Design review of the part built by this model. Coordinates are the model's own, in mm. A direction names the side the tool comes from. Coordinates: 2 decimals unless noted, no trailing zeros. Use a Markdown table: item, result.
from build123d import *

# Parameters (mm, degrees)
F0_R     = 11.1
F0_R_2   = 7
F1_DEPTH = 0.6
F2_DEPTH = 8.5
F3_R     = 11.8527911282
F4_SIZE  = 0.8
F5_DEPTH = 1.3


# Not quite as in the source:
# - a feature names something its author has since deleted; it is built from what else it names


with BuildPart() as f1:
    # F0 (on Top) → F1 (new body)
    with BuildSketch(Plane.XY):
        with BuildLine():
            ThreePointArc((-3.5707142143, 12.5), (0, 13), (3.5707142143, 12.5))
            ThreePointArc((3.5707142143, 12.5), (10.3783256064, 17.1711841504), (13, 25))
            ThreePointArc((13, 25), (-7.8288158496, 35.3783256064), (-3.5707142143, 12.5))
        make_face()
        Polygon((4.9074772881, 33.5), (9.8149545762, 25), (4.9074772881, 16.5), (-4.9074772881, 16.5), (-9.8149545762, 25), (-4.9074772881, 33.5), align=None, mode=Mode.SUBTRACT)
        with BuildLine():
            ThreePointArc((-9.0399604402, -9.3423292192), (-11.2583302492, -6.5), (-12.6106746544, -3.1576707808))
            ThreePointArc((-12.6106746544, -3.1576707808), (-33.6197513051, -17.5734856991), (-8.6506350946, -12.5))
            ThreePointArc((-8.6506350946, -12.5), (-8.7483335459, -10.9092093959), (-9.0399604402, -9.3423292192))
        make_face()
        Polygon((-26.5581123827, -4), (-16.7431578065, -4), (-11.8356805184, -12.5), (-16.7431578065, -21), (-26.5581123827, -21), (-31.4655896708, -12.5), align=None, mode=Mode.SUBTRACT)
        with BuildLine():
            ThreePointArc((34.6506350946, -12.5), (26.7241207937, -0.5308837895), (12.6106746544, -3.1576707808))
            ThreePointArc((12.6106746544, -3.1576707808), (11.2583302492, -6.5), (9.0399604402, -9.3423292192))
            ThreePointArc((9.0399604402, -9.3423292192), (20.0598444905, -25.4023015487), (34.6506350946, -12.5))
        make_face()
        Polygon((16.7431578065, -21), (11.8356805184, -12.5), (16.7431578065, -4), (26.5581123827, -4), (31.4655896708, -12.5), (26.5581123827, -21), align=None, mode=Mode.SUBTRACT)
        with BuildLine():
            ThreePointArc((12.6106746544, -3.1576707808), (12.9023015487, -1.5907906041), (13, 0))
            ThreePointArc((13, 0), (10.3783256064, 7.8288158496), (3.5707142143, 12.5))
            ThreePointArc((3.5707142143, 12.5), (0, 12), (-3.5707142143, 12.5))
            ThreePointArc((-3.5707142143, 12.5), (-11.2583302492, 6.5), (-12.6106746544, -3.1576707808))
            ThreePointArc((-12.6106746544, -3.1576707808), (-10.3923048454, -6), (-9.0399604402, -9.3423292192))
            ThreePointArc((-9.0399604402, -9.3423292192), (0, -13), (9.0399604402, -9.3423292192))
            ThreePointArc((9.0399604402, -9.3423292192), (10.3923048454, -6), (12.6106746544, -3.1576707808))
        make_face()
        Circle(F0_R, mode=Mode.SUBTRACT)
        Circle(F0_R)
        Circle(F0_R_2, mode=Mode.SUBTRACT)
        Polygon((4.9074772881, 16.5), (9.8149545762, 25), (4.9074772881, 33.5), (-4.9074772881, 33.5), (-9.8149545762, 25), (-4.9074772881, 16.5), align=None)
        Polygon((-11.8356805184, -12.5), (-16.7431578065, -4), (-26.5581123827, -4), (-31.4655896708, -12.5), (-26.5581123827, -21), (-16.7431578065, -21), align=None)
        Polygon((16.7431578065, -4), (11.8356805184, -12.5), (16.7431578065, -21), (26.5581123827, -21), (31.4655896708, -12.5), (26.5581123827, -4), align=None)
        with BuildLine():
            ThreePointArc((-3.5707142143, 12.5), (0, 12), (3.5707142143, 12.5))
            ThreePointArc((3.5707142143, 12.5), (0, 13), (-3.5707142143, 12.5))
        make_face()
        with BuildLine():
            ThreePointArc((-9.0399604402, -9.3423292192), (-10.3923048454, -6), (-12.6106746544, -3.1576707808))
            ThreePointArc((-12.6106746544, -3.1576707808), (-11.2583302492, -6.5), (-9.0399604402, -9.3423292192))
        make_face()
        with BuildLine():
            ThreePointArc((9.0399604402, -9.3423292192), (11.2583302492, -6.5), (12.6106746544, -3.1576707808))
            ThreePointArc((12.6106746544, -3.1576707808), (10.3923048454, -6), (9.0399604402, -9.3423292192))
        make_face()
    extrude(amount=F1_DEPTH)

    # F0 (on Top) → F2 (join)
    with BuildSketch(Plane.XY):
        with BuildLine():
            ThreePointArc((-3.5707142143, 12.5), (0, 13), (3.5707142143, 12.5))
            ThreePointArc((3.5707142143, 12.5), (10.3783256064, 17.1711841504), (13, 25))
            ThreePointArc((13, 25), (-7.8288158496, 35.3783256064), (-3.5707142143, 12.5))
        make_face()
        Polygon((4.9074772881, 33.5), (9.8149545762, 25), (4.9074772881, 16.5), (-4.9074772881, 16.5), (-9.8149545762, 25), (-4.9074772881, 33.5), align=None, mode=Mode.SUBTRACT)
        with BuildLine():
            ThreePointArc((12.6106746544, -3.1576707808), (12.9023015487, -1.5907906041), (13, 0))
            ThreePointArc((13, 0), (10.3783256064, 7.8288158496), (3.5707142143, 12.5))
            ThreePointArc((3.5707142143, 12.5), (0, 12), (-3.5707142143, 12.5))
            ThreePointArc((-3.5707142143, 12.5), (-11.2583302492, 6.5), (-12.6106746544, -3.1576707808))
            ThreePointArc((-12.6106746544, -3.1576707808), (-10.3923048454, -6), (-9.0399604402, -9.3423292192))
            ThreePointArc((-9.0399604402, -9.3423292192), (0, -13), (9.0399604402, -9.3423292192))
            ThreePointArc((9.0399604402, -9.3423292192), (10.3923048454, -6), (12.6106746544, -3.1576707808))
        make_face()
        Circle(F0_R, mode=Mode.SUBTRACT)
        with BuildLine():
            ThreePointArc((-3.5707142143, 12.5), (0, 12), (3.5707142143, 12.5))
            ThreePointArc((3.5707142143, 12.5), (0, 13), (-3.5707142143, 12.5))
        make_face()
        with BuildLine():
            ThreePointArc((-9.0399604402, -9.3423292192), (-11.2583302492, -6.5), (-12.6106746544, -3.1576707808))
            ThreePointArc((-12.6106746544, -3.1576707808), (-33.6197513051, -17.5734856991), (-8.6506350946, -12.5))
            ThreePointArc((-8.6506350946, -12.5), (-8.7483335459, -10.9092093959), (-9.0399604402, -9.3423292192))
        make_face()
        Polygon((-26.5581123827, -4), (-16.7431578065, -4), (-11.8356805184, -12.5), (-16.7431578065, -21), (-26.5581123827, -21), (-31.4655896708, -12.5), align=None, mode=Mode.SUBTRACT)
        with BuildLine():
            ThreePointArc((-9.0399604402, -9.3423292192), (-10.3923048454, -6), (-12.6106746544, -3.1576707808))
            ThreePointArc((-12.6106746544, -3.1576707808), (-11.2583302492, -6.5), (-9.0399604402, -9.3423292192))
        make_face()
        with BuildLine():
            ThreePointArc((34.6506350946, -12.5), (26.7241207937, -0.5308837895), (12.6106746544, -3.1576707808))
            ThreePointArc((12.6106746544, -3.1576707808), (11.2583302492, -6.5), (9.0399604402, -9.3423292192))
            ThreePointArc((9.0399604402, -9.3423292192), (20.0598444905, -25.4023015487), (34.6506350946, -12.5))
        make_face()
        Polygon((16.7431578065, -21), (11.8356805184, -12.5), (16.7431578065, -4), (26.5581123827, -4), (31.4655896708, -12.5), (26.5581123827, -21), align=None, mode=Mode.SUBTRACT)
        with BuildLine():
            ThreePointArc((9.0399604402, -9.3423292192), (11.2583302492, -6.5), (12.6106746544, -3.1576707808))
            ThreePointArc((12.6106746544, -3.1576707808), (10.3923048454, -6), (9.0399604402, -9.3423292192))
        make_face()
    extrude(amount=F2_DEPTH)

    # F3
    f3_edges = [f1.edges().sort_by_distance(p)[0] for p in [
        (3.570714, 12.5, 4.25),
        (-3.570714, 12.5, 4.25),
        (-12.610675, -3.157671, 4.25),
        (-9.03996, -9.342329, 4.25),
        (9.03996, -9.342329, 4.25),
        (12.610675, -3.157671, 4.25),
    ]]
    fillet(f3_edges, radius=F3_R)

    # F4
    f4_edges = [f1.edges().sort_by_distance(p)[0] for p in [
        (11.25833, 6.5, 8.5),
        (9.627694, 12.5, 8.5),
        (0, 38, 8.5),
        (-9.627694, 12.5, 8.5),
        (-11.25833, 6.5, 8.5),
        (-11.25833, 6.5, 0),
        (-9.627694, 12.5, 0),
        (0, 38, 0),
        (9.627694, 12.5, 0),
        (11.25833, 6.5, 0),
        (15.639164, 2.087827, 8.5),
        (-15.639164, 2.087827, 8.5),
        (32.908965, -19, 8.5),
        (-32.908965, -19, 8.5),
        (6.011471, -14.587827, 8.5),
        (-6.011471, -14.587827, 8.5),
        (0, -13, 8.5),
        (15.639164, 2.087827, 0),
        (-15.639164, 2.087827, 0),
        (32.908965, -19, 0),
        (-32.908965, -19, 0),
        (6.011471, -14.587827, 0),
        (-6.011471, -14.587827, 0),
        (0, -13, 0),
    ]]
    chamfer(f4_edges, length=F4_SIZE)

    # F0 (on Top) → F5 (join)
    with BuildSketch(Plane.XY):
        Circle(F0_R)
        Circle(F0_R_2, mode=Mode.SUBTRACT)
    extrude(amount=F5_DEPTH)


solid = f1.part
(1) For pin 1 (4 mm diameter, centred on x = 21, z = 3, fed in from +Y); pin 2 (4 mm diameter, centred on x = -19.5, z = 4, fed in from +Y); pin 3 (11 mm diameter, centred on x = -3.5, y = -1, fed in from +Z), all flat-tipped, find the tip position at first contact; note any pin that passes through.
Determined:
| item | result |
|---|---|
| pin 1 | y = 0.78 |
| pin 2 | y = 1.22 |
| pin 3 | z = 1.3 |
(2) Machinability: for faces 3 (the flat face through (-29.046, -8.31, 4.495)), 4 (the conical face through (0.362, 37.334, 0.139)), which of the approach directions +Z, -Z, +X, -X, +Y, -Y give a long, thin tool a straight path to every point of the face, cutting with its end or side? Answer none if there is none.
Determined:
| item | result |
|---|---|
| face 3 | +Z |
| face 4 | -Z |
(3) Draft analysis for pull direction Y (two halves, no side actions). For faces 1 (the conical face through (-32.513, -18.353, 0.139)), 2 (the flat face through (-28.977, -16.81, 4.495)), state which applies: +Y half, -Y half, draft (parallel to the pull), parting line (faces both ways), or undercut.
Determined:
| item | result |
|---|---|
| face 1 | parting line |
| face 2 | undercut |
(4) Take a section at A-A on z = 6.5. State how many separate pieces and enclosed holes the cut face has, and give its area (3 significant figures).
Determined:
| item | result |
|---|---|
| separate pieces | 1 |
| enclosed holes | 4 |
| area | 1,090 mm2 |
(5) For L1, parallel to Y at x = 0, z = 1.05; L2, parallel to Y at x = 0, z = 7; L3, parallel to X at y = -20.5, z = 5, list the stretches that pass through material, from the lowest coordinate up. Write a range as from..to.
Determined:
| item | result |
|---|---|
| L1 | -13..-7, 7..16.5, 33.5..38 |
| L2 | -13..-11.1, 11.1..16.5, 33.5..38 |
| L3 | -31.9..-26.85, -16.45..-11.4, 11.4..16.45, 26.85..31.9 |
